For this review, take the finished solid that the model builds, in its own axes (mm). Coordinates: 2 decimals unless noted, no trailing zeros. Order: outer loops, then holes, each group sorted by start corner. A loop starts at its lowest first (then second) coordinate and runs counter-clockwise, first axis right, second up.
Autodesk Inventor part; units mm, degrees
ref_plane "YZ Plane" through (0, 0, 0) normal (1, 0, 0) x (0, 1, 0)
ref_plane "XZ Plane" through (0, 0, 0) normal (0, 1, 0) x (-1, 0, 0)
ref_plane "XY Plane" through (0, 0, 0) normal (0, 0, 1) x (1, 0, 0)
sketch "Sketch1" plane through (0, 0, 0) normal (0, 0, 1) x (1, 0, 0)
  line L0 (140, 5) -> (-140, 5)
  line L1 (-140, 5) -> (-140, -5)
  line L2 (-140, -5) -> (140, -5)
  line L3 (140, -5) -> (140, 5)
  line L4 (140, 5) -> (-140, -5) construction
  line L5 (-140, 5) -> (140, -5) construction
  point P0 (0, 0)
  dimension "d0" = 280
  dimension "d1" = 10
extrude "Extrusion1" add sketch "Sketch1" along normal blind 20
sketch "Sketch6" plane through (-140, -5, 0) normal (0, -1, 0) x (1, 0, 0)
  line L0 (0, 0) -> (0, 20)
  line L1 (0, 0) -> (280, 0)
  line L2 (0, 20) -> (280, 20)
  line L3 (280, 20) -> (280, 0)
  line L4 (280, 0) -> (0, 0)
  line L5 (0, 0) -> (0, 20)
  point P0 (140, 0)
extrude "Extrusion4" add sketch "Sketch6" along normal blind 3
sketch "Sketch7" plane through (-140, -8, 0) normal (0, -1, 0) x (1, 0, 0)
  point P0 (140, 0)
sketch "Sketch8" plane through (-140, -8, 0) normal (0, -1, 0) x (1, 0, 0)
  circle A0 centre (37.5, 12) radius 2.1
  circle A1 centre (37.5, 12) radius 2.15
  circle A2 centre (233.4451, 12) radius 2.15
  point P0 (140, 0)
  dimension "d23" = 4.3
  dimension "d24" = 4.3
extrude "Extrusion5" cut sketch "Sketch8" against normal through all contours A0 | A1 | A2
sketch "Sketch9" plane through (-140, 5, 0) normal (0, 1, 0) x (1, 0, 0)
  circle A0 centre (37.5, -12) radius 2.15
  circle A1 centre (37.5, -12) radius 3.5
  circle A2 centre (233.4451, -12) radius 2.15
  circle A3 centre (233.4451, -12) radius 3.5
  point P0 (140, 0)
  dimension "d27" = 7
  dimension "d28" = 7
extrude "Extrusion6" cut sketch "Sketch9" against normal blind 10 contours A0 | A1 | A2 | A3
sketch "Sketch10" plane through (-140, 5, 0) normal (-1, 0, 0) x (0, 0, 1)
  line L0 (0, 0) -> (20, 0)
  line L1 (20, 0) -> (20, -10)
  line L2 (20, 0) -> (20, -13)
  line L3 (20, 0) -> (30, 0) construction
  line L4 (0, 0) -> (0, -13)
  line L5 (20, -10) -> (0, 0)
  line L6 (0, 0) -> (20, 0)
  point P0 (0, -5)
  dimension "d31" = 10
  dimension "d32" = 90
extrude "Extrusion7" cut sketch "Sketch10" against normal through all
properties part number "paw shelf_v02"
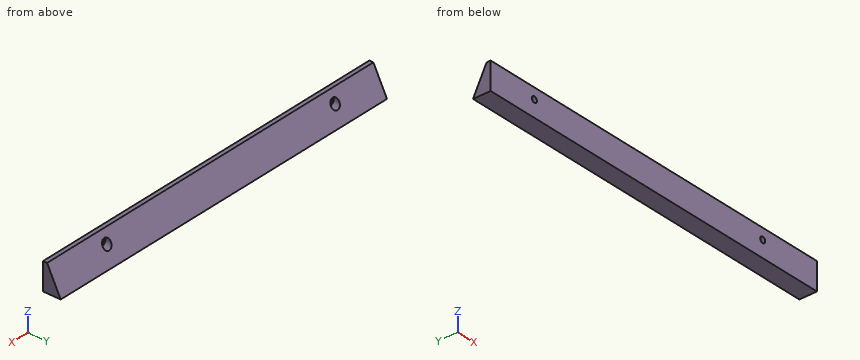
1. Clearance check with flat-ended pins moving along their axes: pin 1 Ø5 at (x, y) = (-50, -1.5) entering from -Z; pin 2 Ø3 at (x, y) = (39, 1) entering from +Z; pin 3 Ø9 at (x, z) = (-102.5, 12) entering from +Y; pin 4 Ø2 at (x, z) = (-101.5, 13) entering from +Y. State where each tip first meets the part, or that it passes through.
Answer below:
pin 1: stops at z = 0
pin 2: stops at z = 11
pin 3: stops at y = 1.25
pin 4: stops at y = -5
2. Take a section at A-A, the plane x = -71. Give the boundary of the cut face in (y, z), plus the area to 3 significant figures.
Answer below:
outline: (-8, 0) - (5, 0) - (-5, 20) - (-8, 20) - close
area: 160 mm2
3. To check wall thickness, follow L1, parallel to X at y = -2.8, z = 12; L2, parallel to X at y = -4.5, z = 14; L3, parallel to Z at x = -102.5, y = -7.2. State the ranges of each line that lie inside material, in increasing order.
Answer below:
L1: x = -140 to -106, -99 to 89.95, 96.95 to 140
L2: x = -140 to -105.37, -99.63 to 90.57, 96.32 to 140
L3: z = 0 to 9.85, 14.15 to 20
